Can you work these out from the drawing? Everything is in mm from the part's minimum corner. A direction names the side the tool comes from. Give positions to 0.01 mm unless a question says otherwise; leave off trailing zeros. Loops run counter-clockwise (first coordinate to the right, second up) from the corner with the lowest first, then second, coordinate; pieces in that order, holes last. Notation, with made-up numbers: M 36.5,34 L 87.5,34 A31 ccw 87.5,62 Z; hole C -35,22 d11. An arc over 180 degrees is marked long. Use CSV: the item, a comma, the result in double quotes.
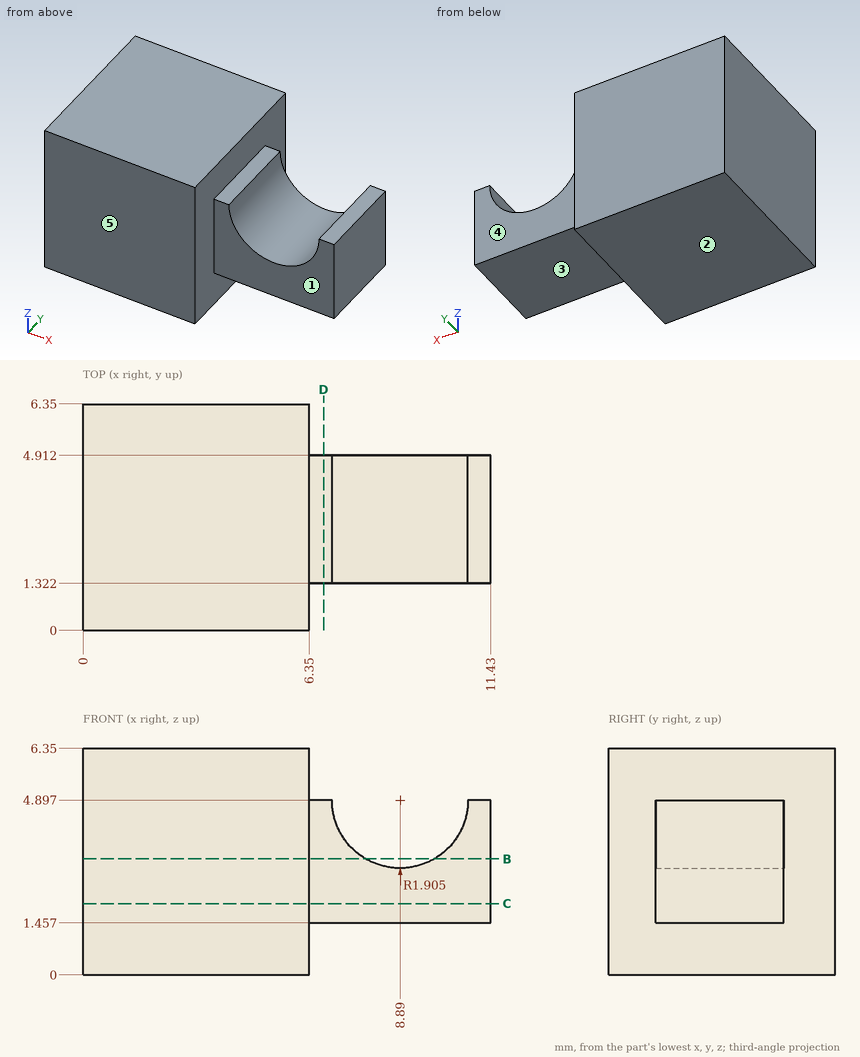
Q1. I want a section at C-C, the plane z = 2. Please give me the cut outline in (x, y).
Model answer:
outline,"M 0,0 L 6.35,0 L 6.35,1.32 L 11.43,1.32 L 11.43,4.91 L 6.35,4.91 L 6.35,6.35 L 0,6.35 Z"
Q2. I want a section at D-D, the plane x = 6.75. Please give me the cut outline in (y, z).
Model answer:
outline,"M 1.32,1.46 L 4.91,1.46 L 4.91,4.9 L 1.32,4.9 Z"
Q3. Please list where these lines run through material, in increasing order: L1, parallel to X at y = 5.25, z = 0.5; L2, parallel to Y at x = 7, z = 4; L3, parallel to X at y = 3, z = 4. Write a range as from..to.
Model answer:
L1,"0..6.35"
L2,"1.32..4.91"
L3,"0..7.21, 10.57..11.43"
Q4. I want a section at B-B, the plane z = 3.25. Please give me the cut outline in (x, y).
Model answer:
outline,"M 0,0 L 6.35,0 L 6.35,1.32 L 7.93,1.32 L 7.93,4.91 L 6.35,4.91 L 6.35,6.35 L 0,6.35 Z; M 9.85,1.32 L 11.43,1.32 L 11.43,4.91 L 9.85,4.91 Z"
Q5. I'm going to push flat-ended pins straight in: P1, Ø0.5, axis at x = 11, y = 4, coming from the +Z side; P2, Ø1.7, axis at x = 10, z = 3, coming from the +Y side; P3, Ø3, axis at x = 8, z = 2.5, coming from the -Y side. Where does each tip first touch, or does it pass through?
Model answer:
P1,"z = 4.9"
P2,"y = 4.91"
P3,"y = 1.32"
Q6. For the marked faces 1, 2, 3, 4 and 5, which set-ups out of +Z, -Z, +X, -X, +Y, -Y let a thin tool reach every point of the face, with its end or its side?
Model answer:
face 1,"+Z, -Z, +X, -Y"
face 2,"-Z, +X, -X, +Y, -Y"
face 3,"-Z, +X, +Y, -Y"
face 4,"+Z, -Z, +X, +Y"
face 5,"+Z, -Z, +X, -X, -Y"
